Job drawing, mm, ordinate dimensions from the low corner. One solid piece. A direction names the side the tool comes from. Round coordinates to 2 decimals unless told otherwise and drop trailing zeros. Loops run counter-clockwise (first coordinate to the right, second up) from the corner with the lowest first, then second, coordinate; pieces in that order, holes last. Notation, with made-up numbers: M -35,8.5 L -6,8.5 A16 cw -6,39.5 Z; hole C -1.5,36.25 d11. An arc over 180 degrees is marked long. Write each question's results on one line, items separated by ' | '. Start each with the question number.
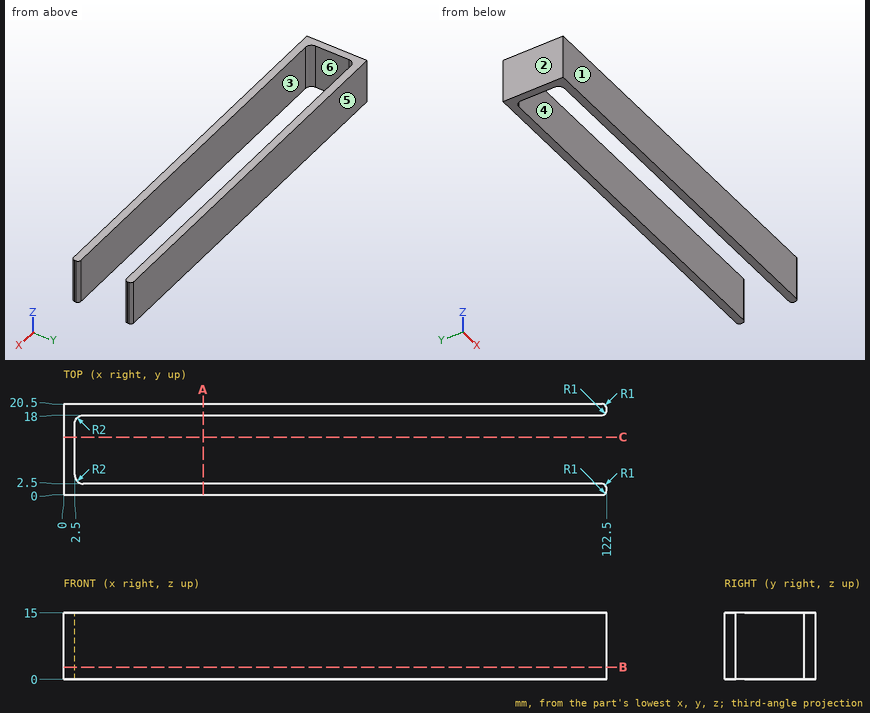
Item 1: Tool access for the marked faces 5 and 6: list every direction of +Z, -Z, +X, -X, +Y, -Y with a clear straight run to the whole face (end or side of a thin tool).
Item 2: Drill centre lines: line 1 along Y through (x, z) = (117, 7.75); line 2 along X through (y, z) = (11.25, 8); line 3 along X through (y, z) = (3.25, 7). Where is each one in solid material? Low to high. Write a range as [from, to].
Item 3: Saw through at C-C, the plane y = 13. Give the cut face in (x, z).
Item 4: Saw through at B-B, the plane z = 2.75. Give the cut face in (x, y), then the cut area to 3 significant figures.
Item 5: Drop flat-ended pins along their axis: pin 1 (3.5 mm diameter, centred on y = 11, z = 4, fed in from +X); pin 2 (8 mm diameter, centred on y = 5, z = 12.5, fed in from -X); pin 3 (1.5 mm diameter, centred on y = 4.5, z = 4.5, fed in from +X); pin 4 (6 mm diameter, centred on x = 30, y = 7, fed in from +Z). Give the stop position or say it passes through.
Item 6: Mould opens along Y. For the marked faces 1, 2, 3 and 4 say: released by +Y, released by -Y, zero draft, split by the parting line, or undercut.
Item 7: Saw through at A-A, the plane x = 31.5. Give the cut face in (y, z), then the cut area to 3 significant figures.
Working result:
1) face 5: +Z, -Z, +X, -X, +Y | face 6: +Z, -Z, +X
2) line 1: y = [0, 2.5], [18, 20.5] | line 2: x = [0, 2.5] | line 3: x = [0, 2.94]
3) outline: M 0,0 L 2.5,0 L 2.5,15 L 0,15 Z
4) outline: M 0,0 L 121.5,0 A1 ccw 122.5,1 L 122.5,1.5 A1 ccw 121.5,2.5 L 4.5,2.5 A2 cw 2.5,4.5 L 2.5,16 A2 cw 4.5,18 L 121.5,18 A1 ccw 122.5,19 L 122.5,19.5 A1 ccw 121.5,20.5 L 0,20.5 Z | area: 652 mm²
5) pin 1: stops at x = 2.5 | pin 2: stops at x = 0 | pin 3: stops at x = 2.65 | pin 4: passes through
6) face 1: released by -Y | face 2: zero draft | face 3: undercut | face 4: undercut
7) outline: M 0,0 L 2.5,0 L 2.5,15 L 0,15 Z; M 18,0 L 20.5,0 L 20.5,15 L 18,15 Z | area: 75.0 mm²
